The model under review builds one solid part; all positions refer to its coordinate system, in mm. A direction names the side the tool comes from. Round coordinates to 2 decimals unless told otherwise and drop trailing zeros. Write each loop counter-clockwise with the first axis right and the second up, starting at its lowest first coordinate (ties: lowest second). Pieces come first, ordered by that corner, then holes. Notation, with made-up numbers: (-19, 1.5) -> (33, 1.5) arc R25 ccw to (33, 36.5) -> close; hole circle Ø5 at (58, 20.5). An arc over 180 degrees is marked (long way). Return JSON: item names as keys, results as strings. Group by question number.
1. Mouldability with a two-part tool opening along Z and no side actions: class faces 1 (the flat face through (175, -36, -2)), 2 (the flat face through (-6, 5, 95)), 3 (the flat face through (112, -5, -150)) as pulls with the +Z half, pulls with the -Z half, needs draft (parallel to the pull), parting line crosses it, or undercut.
2. Take a section at C-C, the plane x = -147.5. Write out the cut boundary in (y, z), then the cut area to 3 significant figures.
3. For line 1 along X through (y, z) = (0.5, 136.5); line 2 along X through (y, z) = (-49.5, -68.5); line 3 along X through (y, z) = (3.6, -121.4), list the stretches that pass through material, from the lowest coordinate up. Write a range as from..to.
4. Take a section at B-B, the plane z = 13.5. Write out the cut boundary in (x, y).
5. Clearance check with flat-ended pins moving along their axes: P1, Ø1, axis at x = 90, z = -66, coming from the -Y side; P2, Ø3, axis at x = -6, y = -42.5, coming from the -Z side; P3, Ø1.5, axis at x = -85, z = 138.5, coming from the +Y side. State where each tip first meets the part, or that it passes through.
6. Take a section at A-A, the plane z = 81.5. Write out the cut boundary in (x, y).
7. Tool access review of faces 4 (the flat face through (-172, -36, -150)), 5 (the flat face through (118, 5, 2)), 6 (the flat face through (170, -39, -5)), 7 (the flat face through (-125, -12, -145)), 8 (the flat face through (3, 7, 53.5)): name each direction out of +Z, -Z, +X, -X, +Y, -Y from which nothing blocks a thin tool from reaching the whole face with its end or side.
Autodesk Inventor part; units mm, degrees
ref_plane "YZ Plane" through (0, 0, 0) normal (1, 0, 0) x (0, 1, 0)
ref_plane "XZ Plane" through (0, 0, 0) normal (0, 1, 0) x (-1, 0, 0)
ref_plane "XY Plane" through (0, 0, 0) normal (0, 0, 1) x (1, 0, 0)
sketch "Sketch2" plane through (0, 0, 0) normal (0, 1, 0) x (-1, 0, 0)
  line L0 (-175, 150) -> (175, 150)
  line L1 (175, 150) -> (175, -150)
  line L2 (175, -150) -> (-175, -150)
  line L3 (-175, -150) -> (-175, 150)
  line L4 (-175, 150) -> (175, -150) construction
  line L5 (175, 150) -> (-175, -150) construction
  point P0 (0, 0)
  dimension "d6" = 350
  dimension "d7" = 300
extrude "Extrusion1" add sketch "Sketch2" along normal blind 10
sketch "Sketch4" plane through (0, 10, 0) normal (0, 1, 0) x (1, 0, 0)
  line L0 (-175, -150) -> (175, -150)
  line L1 (-170, -132.5) -> (-155, -132.5)
  line L2 (-155, -132.5) -> (-155, -105.5)
  line L3 (-155, -105.5) -> (-170, -105.5)
  line L4 (-170, -105.5) -> (-170, -132.5)
  point P0 (0, 0)
  point P1 (-170, -142.5)
  point P2 (-13, -145)
  point P3 (-170, -142.5)
  dimension "d122" = 15
  dimension "d123" = 27
sketch "Sketch5" plane through (0, 10, 0) normal (0, 1, 0) x (1, 0, 0)
  line L0 (-155, -117.5) -> (-155, -142.5)
  line L1 (-175, -150) -> (175, -150)
  line L2 (-13, -137.5) -> (18, -137.5)
  line L3 (18, -137.5) -> (18, -53.5)
  line L4 (18, -53.5) -> (-13, -53.5)
  line L5 (-13, -137.5) -> (-13, -53.5)
  point P0 (0, 0)
  dimension "d24" = 31
  dimension "d25" = 84
extrude "Extrusion3" cut sketch "Sketch5" against normal blind 5
sketch "Sketch7" plane through (0, 10, 0) normal (0, 1, 0) x (1, 0, 0)
  line L0 (-13, -53.5) -> (18, -53.5)
  line L1 (175, 150) -> (-175, 150)
  line L2 (-170, 150) -> (-155, 150)
  line L3 (-155, 150) -> (-155, 136.5)
  line L4 (-155, 136.5) -> (-170, 136.5)
  line L5 (-170, 136.5) -> (-170, 150)
  line L6 (-13, 136.5) -> (2, 136.5)
  line L7 (2, 136.5) -> (2, 150)
  line L8 (2, 150) -> (-13, 150)
  line L9 (-13, 150) -> (-13, 136.5)
  point P0 (0, 0)
  point P1 (-13, -63.5)
  point P2 (-170, -117.5)
  point P3 (-155, 150)
  point P4 (-170, 150)
  dimension "d34" = 15
  dimension "d35" = 13.5
  dimension "d39" = 15
  dimension "d53" = 13.5
extrude "Extrusion6" cut sketch "Sketch7" against normal blind 5
sketch "Sketch8" plane through (0, 5, 0) normal (0, 1, 0) x (1, 0, 0)
  line L0 (2, 150) -> (2, 136.5)
  line L1 (-13, 136.5) -> (-13, 150)
  line L2 (-3.5, 136.5) -> (-7.5, 136.5)
  line L3 (-7.5, 136.5) -> (-7.5, 150)
  line L4 (-7.5, 150) -> (-3.5, 150)
  line L5 (-3.5, 150) -> (-3.5, 136.5)
  line L6 (-3.5, 136.5) -> (-7.5, 150) construction
  line L7 (-7.5, 136.5) -> (-3.5, 150) construction
  line L8 (-170, 136.5) -> (-170, 150)
  line L9 (-170, 143.25) -> (-155, 143.25)
  line L10 (-155, 150) -> (-155, 136.5)
  line L11 (-164.5, 136.5) -> (-160.5, 136.5)
  line L12 (-160.5, 136.5) -> (-160.5, 150)
  line L13 (-160.5, 150) -> (-164.5, 150)
  line L14 (-164.5, 150) -> (-164.5, 136.5)
  line L15 (-164.5, 136.5) -> (-160.5, 150) construction
  line L16 (-160.5, 136.5) -> (-164.5, 150) construction
  point P0 (0, 0)
  point P1 (-5.5, 143.25)
  point P2 (-162.5, 143.25)
  dimension "d42" = 4
  dimension "d43" = 13.5
  dimension "d44" = 4
  dimension "d45" = 13.5
extrude "Extrusion7" cut sketch "Sketch8" against normal through all
sketch "Sketch9" plane through (0, 10, 0) normal (0, 1, 0) x (1, 0, 0)
  point P0 (0, 0)
sketch "Sketch12" plane through (0, 10, 0) normal (0, 1, 0) x (1, 0, 0)
  line L0 (-175, -150) -> (175, -150)
  line L1 (175, -150) -> (175, -145)
  line L2 (175, -150) -> (175, 150)
  line L3 (175, -145) -> (120, -145)
  line L4 (118, 145) -> (122, 145)
  line L5 (122, 145) -> (122, -145)
  line L6 (122, -145) -> (118, -145)
  line L7 (118, -145) -> (118, 145)
  line L8 (118, 145) -> (122, -145) construction
  line L9 (122, 145) -> (118, -145) construction
  point P0 (0, 0)
  point P1 (120, 0)
  dimension "d57" = 5
  dimension "d58" = 55
  dimension "d59" = 4
extrude "Extrusion11" cut sketch "Sketch12" against normal blind 10
sketch "Sketch13" plane through (0, 0, 0) normal (0, -1, 0) x (1, 0, 0)
  line L0 (-175, 150) -> (175, 150)
  line L1 (175, -150) -> (170, -150)
  line L2 (170, -150) -> (170, 150)
  line L3 (170, 150) -> (175, 150)
  line L4 (175, 150) -> (175, -150)
  line L5 (-175, -150) -> (-175, 150)
  line L6 (175, 150) -> (-175, 150)
  line L7 (-175, 150) -> (-175, 145)
  line L8 (-175, 145) -> (175, 145)
  line L9 (175, 145) -> (175, 150)
  line L10 (-175, 150) -> (-170, 150)
  line L11 (-170, 150) -> (-170, -150)
  line L12 (-170, -150) -> (-175, -150)
  line L13 (-175, -150) -> (-175, 150)
  point P0 (0, 0)
  point P1 (175, 150)
  point P2 (-170, 145)
  point P3 (170, 145)
  dimension "d62" = 5
  dimension "d63" = 5
  dimension "d64" = 5
extrude "Extrusion12" add sketch "Sketch13" along normal blind 80
sketch "Sketch14" plane through (0, 10, 0) normal (0, 1, 0) x (1, 0, 0)
  line L0 (2, 150) -> (2, 136.5)
  line L1 (2, 150) -> (19, 150)
  line L2 (170, 150) -> (-3.5, 150)
  line L3 (19, 150) -> (19, 141.9)
  line L4 (19, 141.9) -> (29, 141.9)
  line L5 (29, 141.9) -> (29, 136.9)
  line L6 (29, 136.9) -> (19, 136.9)
  line L7 (19, 136.9) -> (19, 141.9)
  line L8 (19, 123.9) -> (29, 123.9)
  line L9 (29, 123.9) -> (29, 118.9)
  line L10 (29, 118.9) -> (19, 118.9)
  line L11 (19, 118.9) -> (19, 123.9)
  line L12 (19, 121.4) -> (19, 105.9)
  line L13 (19, 105.9) -> (29, 105.9)
  line L14 (29, 105.9) -> (29, 100.9)
  line L15 (29, 100.9) -> (19, 100.9)
  line L16 (19, 100.9) -> (19, 105.9)
  line L17 (-170, 150) -> (-170, -145)
  line L18 (-170, 105.9) -> (-160, 105.9)
  line L19 (-160, 105.9) -> (-160, 100.9)
  line L20 (-160, 100.9) -> (-170, 100.9)
  line L21 (-170, 100.9) -> (-170, 105.9)
  point P0 (0, 0)
  dimension "d67" = 17
  dimension "d68" = 8.1
  dimension "d70" = 5
  dimension "d72" = 5
  dimension "d73" = 15.5
  dimension "d74" = 5
  dimension "d75" = 10
extrude "Extrusion13" cut sketch "Sketch14" against normal blind 5
sketch "Sketch15" plane through (0, 10, 0) normal (0, 1, 0) x (1, 0, 0)
  line L0 (29, 123.9) -> (29, 118.9)
  line L1 (29, 121.4) -> (26.483, 121.4)
  line L2 (29, 105.9) -> (29, 100.9)
  line L3 (29, 103.4) -> (26.483, 103.4)
  line L4 (29, 141.9) -> (29, 136.9)
  line L5 (29, 139.4) -> (26.483, 139.4)
  line L6 (-170, 150) -> (-170, -145)
  line L7 (-170, 103.4) -> (-170, 105.917)
  line L8 (-170, 103.4) -> (-167.483, 103.4)
  point P0 (0, 0)
  dimension "d78" = 2.517
  dimension "d79" = 2.517
  dimension "d80" = 2.517
  dimension "d81" = 2.517
  dimension "d82" = 2.517
hole "Hole1" at (26.483, 10, -139.4) at (26.483, 10, -121.4) at (26.483, 10, -103.4) at (-167.483, 10, -103.4) direction (0, -1, 0) diameter 3.5 end through all
sketch "Sketch16" plane through (0, 0, 0) normal (0, -1, 0) x (1, 0, 0)
  line L0 (170, -150) -> (170, 145)
  line L1 (170, -150) -> (140, -150)
  line L2 (175, -150) -> (2, -150)
  line L3 (140, -150) -> (110, -150)
  line L4 (110, -150) -> (110, -145)
  line L5 (110, -145) -> (140, -145)
  line L6 (140, -145) -> (140, -150)
  line L7 (-170, 145) -> (-170, -150)
  line L8 (-170, -150) -> (-140, -150)
  line L9 (-7.5, -150) -> (-160.5, -150)
  line L10 (-140, -150) -> (-110, -150)
  line L11 (-110, -150) -> (-110, -145)
  line L12 (-110, -145) -> (-140, -145)
  line L13 (-140, -145) -> (-140, -150)
  point P0 (0, 0)
  dimension "d90" = 30
  dimension "d91" = 30
  dimension "d92" = 5
  dimension "d93" = 30
  dimension "d94" = 30
extrude "Extrusion14" add sketch "Sketch16" along normal blind 20
sketch "Sketch17" plane through (-13, 10, -150) normal (0, 0, -1) x (-1, 0, 0)
  line L0 (-153, -10) -> (-153, -30)
  line L1 (-153, -20) -> (-123, -20)
  line L2 (-123, -10) -> (-123, -30)
  line L3 (97, -10) -> (97, -30)
  line L4 (97, -20) -> (127, -20)
  line L5 (127, -10) -> (127, -30)
  point P0 (-13, -10)
  point P1 (-138, -20)
  point P2 (-145.5, -20)
  point P3 (-130.5, -20)
  point P4 (112, -20)
  point P5 (104.5, -20)
  point P6 (119.5, -20)
hole "Hole2" at (-132.5, -10, -150) at (-125, -10, -150) at (-117.5, -10, -150) at (117.5, -10, -150) at (125, -10, -150) at (132.5, -10, -150) direction (0, 0, 1) diameter 3.5 depth 5
sketch "Sketch18" plane through (-175, 10, 150) normal (0, 0, 1) x (1, 0, 0)
  line L0 (350, -90) -> (350, 0)
  line L1 (350, 0) -> (300, 0)
  line L2 (0, 0) -> (350, 0)
  line L3 (300, 0) -> (300, -70)
  line L4 (0, 0) -> (50, 0)
  line L5 (50, 0) -> (50, -70)
  point P0 (175, -10)
  point P1 (292.5, -40)
  point P2 (307.5, -40)
  point P3 (57.5, -40)
  point P4 (42.5, -40)
  dimension "d104" = 50
  dimension "d105" = 70
  dimension "d106" = 50
  dimension "d107" = 70
hole "Hole4" at (-132.5, -30, 150) at (-117.5, -30, 150) at (-125, -60, 150) at (132.5, -30, 150) at (117.5, -30, 150) at (125, -60, 150) direction (0, 0, -1) diameter 3.5 depth 5
extrude "Extrusion15" cut sketch "Sketch4" against normal blind 5
sketch "Sketch19" plane through (0, 10, 0) normal (0, 1, 0) x (1, 0, 0)
  line L0 (-170, -132.5) -> (-170, -105.5)
  line L1 (-170, -119) -> (-155, -119)
  line L2 (-155, -105.5) -> (-155, -132.5)
  line L3 (-170, -105.5) -> (-155, -105.5)
  line L4 (-164.5, -132.5) -> (-160.5, -132.5)
  line L5 (-160.5, -132.5) -> (-160.5, -105.5)
  line L6 (-160.5, -105.5) -> (-164.5, -105.5)
  line L7 (-164.5, -105.5) -> (-164.5, -132.5)
  line L8 (-164.5, -132.5) -> (-160.5, -105.5) construction
  line L9 (-160.5, -132.5) -> (-164.5, -105.5) construction
  point P0 (0, 0)
  point P1 (-162.5, -119)
  dimension "d126" = 4
extrude "Extrusion16" cut sketch "Sketch19" against normal blind 10 contours L7 L3 L5 L1 | L1 L5 L4 L7
sketch "Sketch20" plane through (0, 10, 0) normal (0, 1, 0) x (1, 0, 0)
  line L0 (-13, -137.5) -> (-13, -53.5)
  line L1 (-13, -53.5) -> (18, -53.5)
  line L2 (4.5, -137.5) -> (0.5, -137.5)
  line L3 (0.5, -137.5) -> (0.5, -53.5)
  line L4 (0.5, -53.5) -> (4.5, -53.5)
  line L5 (4.5, -53.5) -> (4.5, -137.5)
  line L6 (4.5, -137.5) -> (0.5, -53.5) construction
  line L7 (0.5, -137.5) -> (4.5, -53.5) construction
  point P0 (0, 0)
  point P1 (2.5, -95.5)
  dimension "d129" = 4
extrude "Extrusion17" cut sketch "Sketch20" against normal blind 10
sketch "Sketch21" plane through (0, 10, 0) normal (0, 1, 0) x (1, 0, 0)
  line L0 (18, -137.5) -> (-13, -137.5)
  line L1 (-13, -137.5) -> (-155, -137.5)
  line L2 (-84, -137.5) -> (-84, -142.5)
  line L3 (-74, -147.5) -> (-94, -147.5)
  line L4 (-94, -147.5) -> (-94, -137.5)
  line L5 (-94, -137.5) -> (-74, -137.5)
  line L6 (-74, -137.5) -> (-74, -147.5)
  line L7 (-74, -147.5) -> (-94, -137.5) construction
  line L8 (-94, -147.5) -> (-74, -137.5) construction
  point P0 (0, 0)
  dimension "d132" = 5
  dimension "d133" = 20
extrude "Extrusion18" cut sketch "Sketch21" against normal blind 5
sketch "Sketch22" plane through (0, 10, 0) normal (0, 1, 0) x (1, 0, 0)
  line L0 (-94, -147.5) -> (-94, -137.5)
  line L1 (-94, -142.5) -> (-74, -142.5)
  line L2 (-74, -137.5) -> (-74, -147.5)
  line L3 (-74, -144.5) -> (-94, -144.5)
  line L4 (-94, -144.5) -> (-94, -140.5)
  line L5 (-94, -140.5) -> (-74, -140.5)
  line L6 (-74, -140.5) -> (-74, -144.5)
  line L7 (-74, -144.5) -> (-94, -140.5) construction
  line L8 (-94, -144.5) -> (-74, -140.5) construction
  point P0 (0, 0)
  point P1 (-84, -142.5)
  dimension "d136" = 4
extrude "Extrusion19" cut sketch "Sketch22" against normal blind 10
properties part number "Venstre"
Output:
{
 "1": {"face 1": "needs draft", "face 2": "undercut", "face 3": "pulls with the -Z half"},
 "2": {"outline": "(-80, 145) -> (0, 145) -> (0, -150) -> (10, -150) -> (10, 150) -> (-80, 150) -> close", "area": "3,400 mm^2"},
 "3": {"line 1": "x = -175..0.5, 4.5..118, 122..175", "line 2": "x = -175..-170, 170..175", "line 3": "x = -175..24.73, 28.23..118, 122..175"},
 "4": {"outline": "(-175, -80) -> (-170, -80) -> (-170, 0) -> (118, 0) -> (118, 10) -> (-175, 10) -> close; (122, 0) -> (170, 0) -> (170, -80) -> (175, -80) -> (175, 10) -> (122, 10) -> close"},
 "5": {"P1": "stops at y = 0", "P2": "stops at z = 145", "P3": "stops at y = 5"},
 "6": {"outline": "(-175, -80) -> (-170, -80) -> (-170, 0) -> (0.5, 0) -> (0.5, 5) -> (-13, 5) -> (-13, 10) -> (-175, 10) -> close; (4.5, 0) -> (118, 0) -> (118, 10) -> (18, 10) -> (18, 5) -> (4.5, 5) -> close; (122, 0) -> (170, 0) -> (170, -80) -> (175, -80) -> (175, 10) -> (122, 10) -> close"},
 "7": {"face 4": "-Z, +X, -X, +Y, -Y", "face 5": "+Y, -Y", "face 6": "-Z, -Y", "face 7": "-Y", "face 8": "+Y"}
}
